Geometry: final body of the model. Coordinates: model frame, mm. Round coordinates to 2 decimals unless told otherwise and drop trailing zeros. Order: outer loops, then holes, each group sorted by start corner. A loop starts at its lowest first (then second) coordinate and runs counter-clockwise, first axis right, second up. Notation, with made-up numbers: (-19, 30.5) - (1, 30.5) arc R16 ccw to (1, 56.5) - close; hole circle Ø11 at (-37.5, 3). An arc over 180 degrees is marked (long way). Put each result on its own line as item: value. Start each with the question number.
(1) Section B-B (x = 373.5). Output: boundary loops of the cut face in (y, z).
(2) Material intervals for L1, parallel to X at y = -18, z = 0; L2, parallel to Y at x = 1430, z = 5.5; L3, parallel to Y at x = 1641.5, z = 15 (1 decimal), sorted ascending. Write a range as [from, to].
(3) Pin query (flat end, axial travel): P1, Ø8, axis at y = -1, z = -11.5, coming from the -X side. Return the tip coordinate at first contact, or that it passes through.
(4) Section A-A (z = 0). Output: boundary loops of the cut face in (x, y), and give its area (3 significant figures).
from build123d import *

# Parameters (mm, degrees)
TUBE_SQUARE_40_X_40_X_3_2_4_DEPTH = 1920
SKETCH13_R                        = 11
CUT_EXTRUDE1_DEPTH                = 1921.52076271


with BuildPart() as part:
    # Sketch12 → Tube (square) 40 X 40 X 3.2(4) (new body)
    with BuildSketch(Plane(origin=(0, 0, 0), x_dir=(0, 0, -1), z_dir=(1, 0, 0))):
        with BuildLine():
            Line((-13.6, -20), (13.6, -20))
            ThreePointArc((13.6, -20), (18.1254834, -18.1254834), (20, -13.6))
            Line((20, -13.6), (20, 13.6))
            ThreePointArc((20, 13.6), (18.1254834, 18.1254834), (13.6, 20))
            Line((13.6, 20), (-13.6, 20))
            ThreePointArc((-13.6, 20), (-18.1254834, 18.1254834), (-20, 13.6))
            Line((-20, 13.6), (-20, -13.6))
            ThreePointArc((-20, -13.6), (-18.1254834, -18.1254834), (-13.6, -20))
        make_face()
        with BuildLine():
            Line((-13.6, -16.8), (13.6, -16.8))
            ThreePointArc((13.6, -16.8), (15.8627417, -15.8627417), (16.8, -13.6))
            Line((16.8, -13.6), (16.8, 13.6))
            ThreePointArc((16.8, 13.6), (15.8627417, 15.8627417), (13.6, 16.8))
            Line((13.6, 16.8), (-13.6, 16.8))
            ThreePointArc((-13.6, 16.8), (-15.8627417, 15.8627417), (-16.8, 13.6))
            Line((-16.8, 13.6), (-16.8, -13.6))
            ThreePointArc((-16.8, -13.6), (-15.8627417, -15.8627417), (-13.6, -16.8))
        make_face(mode=Mode.SUBTRACT)
    extrude(amount=TUBE_SQUARE_40_X_40_X_3_2_4_DEPTH)

    # Sketch13 → Cut-Extrude1 (cut, through all)
    with BuildSketch(Plane(origin=(0, 20, 0), x_dir=(1, 0, 0), z_dir=(0, 1, 0))):
        with Locations(Location((960, 0, 0), (0, 0, 270))):
            Circle(SKETCH13_R)
    extrude(amount=-CUT_EXTRUDE1_DEPTH, mode=Mode.SUBTRACT)


solid = part.part
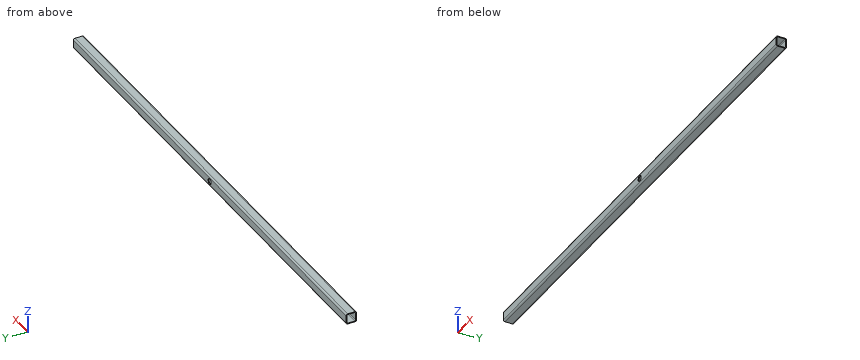
Checks:
1. outline: (-20, -13.6) arc R6.4 ccw to (-13.6, -20) - (13.6, -20) arc R6.4 ccw to (20, -13.6) - (20, 13.6) arc R6.4 ccw to (13.6, 20) - (-13.6, 20) arc R6.4 ccw to (-20, 13.6) - close; hole (-16.8, -13.6) arc R3.2 ccw to (-13.6, -16.8) - (13.6, -16.8) arc R3.2 ccw to (16.8, -13.6) - (16.8, 13.6) arc R3.2 ccw to (13.6, 16.8) - (-13.6, 16.8) arc R3.2 ccw to (-16.8, 13.6) - close
2. L1: x = [0, 949], [971, 1920]
2. L2: y = [-20, -16.8], [16.8, 20]
2. L3: y = [-19.8, -16.5], [16.5, 19.8]
3. P1: passes through
4. outline: (0, -20) - (949, -20) - (949, -16.8) - (0, -16.8) - close; (0, 16.8) - (949, 16.8) - (949, 20) - (0, 20) - close; (971, -20) - (1920, -20) - (1920, -16.8) - (971, -16.8) - close; (971, 16.8) - (1920, 16.8) - (1920, 20) - (971, 20) - close
4. area: 12,100 mm²
